from build123d import *

# Parameters (mm, degrees)
SKETCH_1_R                  = 4.36
EXTRUDE_1_DEPTH             = 5
HOLE_WIZARD_1_5_1_5_1_D     = 4
HOLE_WIZARD_1_5_1_5_1_DEPTH = 2.5
HOLE_WIZARD_1_5_1_5_1_TIP   = 1.154700538
CUT_EXTRUDE_1_DEPTH         = 2.5
SKETCH_4_R                  = 2.5
EXTRUDE_2_DEPTH             = 12
CHAMFER_1_SIZE              = 0.4
FILLET_1_R                  = 0.25


with BuildPart() as part:
    # 草圖1 → 伸長1 (new body)
    with BuildSketch(Plane(origin=(0, 0, 0), x_dir=(0, 0, -1), z_dir=(1, 0, 0))):
        Circle(SKETCH_1_R)
    extrude(amount=-EXTRUDE_1_DEPTH)

    # Ø1.5 (1.5) 直徑孔1
    with Locations(Plane(origin=(-5, 0, 0), x_dir=(0, 0, -1), z_dir=(-1, 0, 0))):
        with Locations((0, 0)):
            Hole(HOLE_WIZARD_1_5_1_5_1_D / 2, depth=HOLE_WIZARD_1_5_1_5_1_DEPTH)
            with Locations((0, 0, -(HOLE_WIZARD_1_5_1_5_1_DEPTH + HOLE_WIZARD_1_5_1_5_1_TIP / 2))):  # 120° drill point
                Cone(0, HOLE_WIZARD_1_5_1_5_1_D / 2, HOLE_WIZARD_1_5_1_5_1_TIP, mode=Mode.SUBTRACT)

    # 草圖3 → 除料-伸長1 (cut)
    with BuildSketch(Plane.ZY.offset(5)):
        Polygon((2.29, 0), (1.145, 1.983198175), (-1.145, 1.983198175), (-2.29, 0), (-1.145, -1.983198175), (1.145, -1.983198175), align=None)
    extrude(amount=-CUT_EXTRUDE_1_DEPTH, mode=Mode.SUBTRACT)

    # 草圖4 → 伸長2 (add)
    with BuildSketch(Plane(origin=(0, 0, 0), x_dir=(0, 0, -1), z_dir=(1, 0, 0))):
        Circle(SKETCH_4_R)
    extrude(amount=EXTRUDE_2_DEPTH)

    # 導角1
    chamfer_1_edges = [part.edges().sort_by_distance(p)[0] for p in [
        (0, 0, 4.36),
        (-5, 0, 4.36),
        (0, 0, 2.5),
        (12, 0, 2.5),
    ]]
    chamfer(chamfer_1_edges, length=CHAMFER_1_SIZE)

    # 圓角1
    fillet_1_edges = [part.edges().sort_by_distance(p)[0] for p in [
        (0.4, 0, 2.5),
        (0, 0, 2.9),
    ]]
    fillet(fillet_1_edges, radius=FILLET_1_R)


solid = part.part
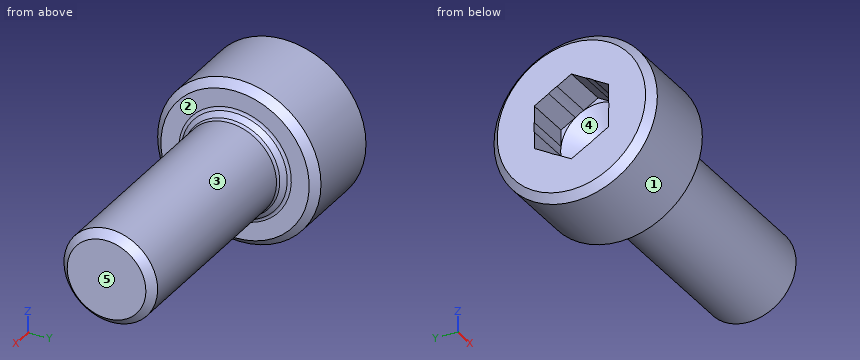
The model under review builds one solid part; all positions refer to its coordinate system, in mm. Face numbers are marked on the shaded views. A direction names the side the tool comes from. Round coordinates to 2 decimals unless told otherwise and drop trailing zeros. Write each loop counter-clockwise with the first axis right and the second up, starting at its lowest first coordinate (ties: lowest second). Pieces come first, ordered by that corner, then holes. Notation, with made-up numbers: M -27.5,63.25 L 10.5,63.25 A27 ccw 10.5,90.25 Z; hole C 38.5,6 d11. An arc over 180 degrees is marked long. Use a Markdown table: item, result. Add a question column.
Q1. The part is to be moulded in two halves that separate along Z. For the marked faces 3, 4 and 5, say which applies: pulls with the +Z half, pulls with the -Z half, needs draft (parallel to the pull), parting line crosses it, or undercut.
Q2. We need section A-A, the plane x = 8.5. State the section outline as (y, z) points.
Q3. Insertion check: pin 1 (1.5 mm diameter, centred on x = 10, z = -0.5, fed in from -Y); pin 2 (0.7 mm diameter, centred on x = -3.5, z = 0.5, fed in from -Y); pin 3 (5 mm diameter, centred on x = 5.5, y = 1, fed in from +Z); pin 4 (0.8 mm diameter, centred on y = -1.5, z = -1, fed in from -X). Each pin has a flat end and moves straight along its axis. Give the tip position at first contact, or say it passes through.
Q4. To check wall thickness, follow line 1 (Y direction, x = 2, z = 0); line 2 (Z direction, x = 11.25, y = 1); line 3 (X direction, y = -2, z = 2.25). State the ranges of each line that lie inside material, in increasing order.
Q5. Machinability: for the marked faces 1 and 2, which of the approach directions +Z, -Z, +X, -X, +Y, -Y give a long, thin tool a straight path to every point of the face, cutting with its end or side? Answer none if there is none.
Findings below:
| question | item | result |
|---|---|---|
| 1 | face 3 | parting line crosses it |
| 1 | face 4 | undercut |
| 1 | face 5 | needs draft |
| 2 | outline | C 0,0 d5 |
| 3 | pin 1 | stops at y = -2.5 |
| 3 | pin 2 | stops at y = -4.36 |
| 3 | pin 3 | stops at z = 2.5 |
| 3 | pin 4 | stops at x = -5 |
| 4 | line 1 | y = -2.5 to 2.5 |
| 4 | line 2 | z = -2.29 to 2.29 |
| 4 | line 3 | x = -5 to 0 |
| 5 | face 1 | +X, -X |
| 5 | face 2 | +X |
